Here's how the part is built. I have some questions about the finished solid (model axes, mm). Face numbers are marked on the shaded views. A direction names the side the tool comes from. Round coordinates to 2 decimals unless told otherwise and drop trailing zeros. Order: outer loops, then holes, each group sorted by start corner. A loop starts at its lowest first (then second) coordinate and runs counter-clockwise, first axis right, second up. Notation, with made-up numbers: (42, 19.5) -> (75, 19.5) arc R33 ccw to (75, 58.5) -> close; hole circle Ø3 at (43.5, -35.75). An arc over 180 degrees is marked (long way). One line per item, written item: value.
```python
from build123d import *

# Parameters (mm, degrees)
ESQUISSE1_W                  = 55
ESQUISSE1_H                  = 75
BOSS_EXTRU_1_DEPTH           = 2
ESQUISSE2_W                  = 2.002378602
ESQUISSE2_H                  = 75
BOSS_EXTRU_2_DEPTH           = 15
CONG_1_R                     = 3
CONG_2_R                     = 10
ENL_V_MAT_EXTRU_1_DEPTH      = 10
ENL_V_MAT_EXTRU_1_DEPTH_BACK = 83.194496151
ESQUISSE6_R                  = 3


# Read off the part's stored shape, not the designer's step: Fraisage pour vis à tête fraisée M61
with BuildPart() as part:
    # Esquisse1 → Boss.-Extru.1 (new body)
    with BuildSketch(Plane.XY):
        with Locations((27.5, 37.5)):
            Rectangle(ESQUISSE1_W, ESQUISSE1_H)
    extrude(amount=BOSS_EXTRU_1_DEPTH)

    # Esquisse2 → Boss.-Extru.2 (add)
    with BuildSketch(Plane.XY.offset(2)):
        with Locations((30.017308917, 37.5)):
            Rectangle(ESQUISSE2_W, ESQUISSE2_H)
        with Locations((24.982691083, 37.5)):
            Rectangle(ESQUISSE2_W, ESQUISSE2_H)
    extrude(amount=BOSS_EXTRU_2_DEPTH)

    # Congé1
    cong_1_edges = [part.edges().sort_by_distance(p)[0] for p in [
        (0, 75, 1),
        (55, 75, 1),
        (55, 0, 1),
        (0, 0, 1),
    ]]
    fillet(cong_1_edges, radius=CONG_1_R)

    # Congé2
    cong_2_edges = [part.edges().sort_by_distance(p)[0] for p in [
        (24.982691083, 75, 17),
        (24.982691083, 0, 17),
        (30.017308917, 0, 17),
        (30.017308917, 75, 17),
    ]]
    fillet(cong_2_edges, radius=CONG_2_R)

    # Fraisage pour vis à tête fraisée M61 out → Fraisage pour vis à tête fraisée M61 (revolve, cut)
    with BuildSketch(Plane(origin=(45.511606252, 65, 0), x_dir=(1, 0, 0), z_dir=(0, -1, 0))):
        Polygon((6.3, 2), (0, 2), (0, 0), (4.3, 0), align=None)
    revolve(axis=Axis((45.511606252, 65, 0), (0, 0, 1)), mode=Mode.SUBTRACT)

    # Fraisage pour vis _ t_te frais_e M61 2 o → Fraisage pour vis _ t_te frais_e M61 2 (revolve, cut)
    with BuildSketch(Plane(origin=(45.511606252, 10, 0), x_dir=(1, 0, 0), z_dir=(0, -1, 0))):
        Polygon((6.3, 2), (0, 2), (0, 0), (4.3, 0), align=None)
    revolve(axis=Axis((45.511606252, 10, 0), (0, 0, 1)), mode=Mode.SUBTRACT)

    # Fraisage pour vis _ t_te frais_e M61 3 o → Fraisage pour vis _ t_te frais_e M61 3 (revolve, cut)
    with BuildSketch(Plane(origin=(9.488393748, 10, 0), x_dir=(1, 0, 0), z_dir=(0, -1, 0))):
        Polygon((6.3, 2), (0, 2), (0, 0), (4.3, 0), align=None)
    revolve(axis=Axis((9.488393748, 10, 0), (0, 0, 1)), mode=Mode.SUBTRACT)

    # Fraisage pour vis _ t_te frais_e M61 4 o → Fraisage pour vis _ t_te frais_e M61 4 (revolve, cut)
    with BuildSketch(Plane(origin=(9.488393748, 65, 0), x_dir=(1, 0, 0), z_dir=(0, -1, 0))):
        Polygon((6.3, 2), (0, 2), (0, 0), (4.3, 0), align=None)
    revolve(axis=Axis((9.488393748, 65, 0), (0, 0, 1)), mode=Mode.SUBTRACT)

    # Esquisse6 → Enlèv. mat.-Extru.1 (cut, two sides: drawn at the far end of the back side and taken through both)
    with BuildSketch(Plane(origin=(25.983880384, 0, 0), x_dir=(0, 0, -1), z_dir=(1, 0, 0)).offset(-ENL_V_MAT_EXTRU_1_DEPTH_BACK)):
        with Locations(Location((-9.133710771, 62.312214024, 0), (0, 0, 270))):
            Circle(ESQUISSE6_R)
        with Locations(Location((-9.133710771, 12.687785976, 0), (0, 0, 270))):
            Circle(ESQUISSE6_R)
    extrude(amount=ENL_V_MAT_EXTRU_1_DEPTH + ENL_V_MAT_EXTRU_1_DEPTH_BACK, mode=Mode.SUBTRACT)


solid = part.part
```
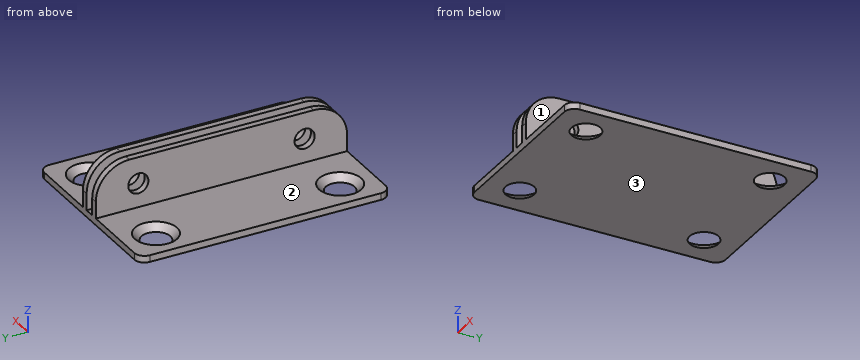
Q1. I want a section at B-B on y = 24. Write out the boundary of the cut face in (x, z).
Answers:
outline: (0, 0) -> (55, 0) -> (55, 2) -> (31.02, 2) -> (31.02, 17) -> (29.02, 17) -> (29.02, 2) -> (25.98, 2) -> (25.98, 17) -> (23.98, 17) -> (23.98, 2) -> (0, 2) -> close
Q2. For P1, Ø10, axis at x = 6.5, z = 8.5, coming from the +Y side; P2, Ø5, axis at x = 28.5, z = 10.5, coming from the +Y side; P3, Ø1.5, axis at y = 8.5, z = 11.5, coming from the -X side; P4, Ø0.9, axis at x = 27, y = 41.5, coming from the +Z side, each with a flat end and sliding along its axis, tell me the tip position at first contact or that it passes through.
Answers:
P1: through
P2: y = 74.94
P3: x = 23.98
P4: z = 2
Q3. I want a section at C-C on x = 33. Write out the boundary of the cut face in (y, z), then the cut area to 3 significant figures.
Answers:
outline: (0, 0) -> (75, 0) -> (75, 2) -> (0, 2) -> close
area: 150 mm2
Q4. Which directions (+Z, -Z, +X, -X, +Y, -Y) give clear straight access to the entire face, cutting with the end or side of a thin tool? Please do the marked faces 1, 2 and 3.
Answers:
face 1: +Z, +X, +Y, -Y
face 2: +Z, -X, +Y, -Y
face 3: -Z, +X, -X, +Y, -Y
Q5. I want a section at D-D on z = 15.75. Write out the boundary of the cut face in (x, y).
Answers:
outline: (23.98, 5.16) -> (25.98, 5.16) -> (25.98, 69.84) -> (23.98, 69.84) -> close; (29.02, 5.16) -> (31.02, 5.16) -> (31.02, 69.84) -> (29.02, 69.84) -> close
Q6. I want a section at A-A on z = 4.25. Write out the boundary of the cut face in (x, y).
Answers:
outline: (23.98, 0) -> (25.98, 0) -> (25.98, 75) -> (23.98, 75) -> close; (29.02, 0) -> (31.02, 0) -> (31.02, 75) -> (29.02, 75) -> close
Q7. I need wall thicknesses on line 1 along X through (y, z) = (52, 3.75); line 2 along Z through (x, y) = (18.5, 25); line 3 along Y through (x, z) = (25.5, 15.75). Which ranges of each line are inside material? Lowest first, please.
Answers:
line 1: 23.98 to 25.98, 29.02 to 31.02
line 2: 0 to 2
line 3: 5.16 to 69.84
